from build123d import *

# Parameters (mm, degrees)
BOSS_EXTRUDE1_DEPTH = 58
SKETCH3_R           = 7.5
CUT_EXTRUDE1_DEPTH  = 107.60206377
CUT_EXTRUDE2_DEPTH  = 107.60206377
CUT_EXTRUDE3_DEPTH  = 107.60206377
SKETCH6_R           = 7
CUT_EXTRUDE4_DEPTH  = 107.60206377
CUT_EXTRUDE5_DEPTH  = 6
CUT_EXTRUDE6_DEPTH  = 4
CUT_EXTRUDE7_START  = -6
CUT_EXTRUDE7_DEPTH  = 6
CUT_EXTRUDE8_START  = -4
CUT_EXTRUDE8_DEPTH  = 4


with BuildPart() as part:
    # Sketch2 → Boss-Extrude1 (new body)
    with BuildSketch(Plane.XY):
        with BuildLine():
            Line((0, 0), (65, 0))
            Line((65, 0), (80, 9.029262631))
            Line((80, 9.029262631), (80, 31.339745962))
            Line((80, 31.339745962), (65, 40))
            Line((65, 40), (36.66060556, 40))
            ThreePointArc((36.66060556, 40), (16.66060556, 35.82575695), (0, 24))
            Line((0, 24), (0, 0))
        make_face()
    extrude(amount=-BOSS_EXTRUDE1_DEPTH)

    # Sketch3 → Cut-Extrude1 (cut, through all)
    with BuildSketch(Plane.XY):
        with Locations((34, 19)):
            Circle(SKETCH3_R)
    extrude(amount=-CUT_EXTRUDE1_DEPTH, mode=Mode.SUBTRACT)

    # Sketch4 → Cut-Extrude2 (cut, through all)
    with BuildSketch(Plane(origin=(0, 0, 0), x_dir=(1, 0, 0), z_dir=(0, 1, 0))):
        Polygon((65, 58), (80, 43), (80, 58), align=None)
        Polygon((80, 0), (80, 15), (65, 0), align=None)
    extrude(amount=CUT_EXTRUDE2_DEPTH, mode=Mode.SUBTRACT)

    # Sketch5 → Cut-Extrude3 (cut, through all)
    with BuildSketch(Plane.XZ):
        Polygon((0, -8), (0, -50), (16, -50), (16, -44), (54, -44), (54, -14), (16, -14), (16, -8), align=None)
    extrude(amount=-CUT_EXTRUDE3_DEPTH, mode=Mode.SUBTRACT)

    # Sketch6 → Cut-Extrude4 (cut, through all)
    with BuildSketch(Plane(origin=(80, 0, 0), x_dir=(0, 0, -1), z_dir=(1, 0, 0))):
        with Locations((29, 20)):
            Circle(SKETCH6_R)
    extrude(amount=-CUT_EXTRUDE4_DEPTH, mode=Mode.SUBTRACT)

    # Sketch8 → Cut-Extrude5 (cut)
    with BuildSketch(Plane.XY):
        with BuildLine():
            Line((1.466424222, 22.64), (0, 21.058823529))
            Line((0, 21.058823529), (0, 2))
            Line((0, 2), (63, 2))
            Line((63, 2), (63, 38))
            Line((63, 38), (36.66060556, 38))
            ThreePointArc((36.66060556, 38), (17.46060556, 33.992726672), (1.466424222, 22.64))
        make_face()
    extrude(amount=-CUT_EXTRUDE5_DEPTH, mode=Mode.SUBTRACT)

    # Sketch9 → Cut-Extrude6 (cut)
    with BuildSketch(Plane.XY.offset(-6)):
        with BuildLine():
            Line((18, 2), (63, 2))
            Line((63, 2), (63, 38))
            Line((63, 38), (36.66060556, 38))
            ThreePointArc((36.66060556, 38), (27.141221384, 37.046586751), (18, 34.224221872))
            Line((18, 34.224221872), (18, 2))
        make_face()
    extrude(amount=-CUT_EXTRUDE6_DEPTH, mode=Mode.SUBTRACT)

    # Sketch10 → Cut-Extrude7 (cut)
    with BuildSketch(Plane(origin=(0, 0, -58), x_dir=(-1, 0, 0), z_dir=(0, 0, -1)).offset(CUT_EXTRUDE7_START)):
        with BuildLine():
            Line((-1.466424222, 22.64), (0, 21.058823529))
            Line((0, 21.058823529), (0, 2))
            Line((0, 2), (-63, 2))
            Line((-63, 2), (-63, 38))
            Line((-63, 38), (-36.66060556, 38))
            ThreePointArc((-36.66060556, 38), (-17.46060556, 33.992726672), (-1.466424222, 22.64))
        make_face()
    extrude(amount=CUT_EXTRUDE7_DEPTH, mode=Mode.SUBTRACT)

    # Sketch11 → Cut-Extrude8 (cut)
    with BuildSketch(Plane(origin=(0, 0, -52), x_dir=(-1, 0, 0), z_dir=(0, 0, -1)).offset(CUT_EXTRUDE8_START)):
        with BuildLine():
            Line((-63, 38), (-63, 2))
            Line((-63, 2), (-18, 2))
            Line((-18, 2), (-18, 34.224221872))
            ThreePointArc((-18, 34.224221872), (-27.141221384, 37.046586751), (-36.66060556, 38))
            Line((-36.66060556, 38), (-63, 38))
        make_face()
    extrude(amount=CUT_EXTRUDE8_DEPTH, mode=Mode.SUBTRACT)


solid = part.part
Input: part model. Units: mm. Frame: model coordinates. A direction names the side the tool comes from. Coordinates: 2 decimals unless noted, no trailing zeros. Order: outer loops, then holes, each group sorted by start corner. A loop starts at its lowest first (then second) coordinate and runs counter-clockwise, first axis right, second up. Notation, with made-up numbers: M 63.5,41.5 L 122.5,41.5 A13 cw 122.5,53.5 Z; hole C 73,-34.75 d9. An arc over 180 degrees is marked long. One line per question, with ' | ' between items.
Item 1: Section D-D (y = 20). Give the number of separate pieces and of enclosed holes in the cut face, then the cut area to 3 significant figures.
Geometry results:
separate pieces: 4 | enclosed holes: 0 | area: 1,000 mm^2
Item 2: Draft query along X for faces 6 (the flat face through (9, 15, -52)), 7 (the flat face through (70.94, 36.57, -28.59)), 8 (the flat face through (38, 2, -5)), 9 (the flat face through (44, 20, -14)). Return one class per face: released by +X, released by -X, zero draft, split by the parting line, or undercut.
Geometry results:
face 6: undercut | face 7: released by +X | face 8: undercut | face 9: zero draft
Item 3: Section C-C (x = 51). Output: boundary loops of the cut face in (y, z), then the cut area to 3 significant figures.
Geometry results:
outline: M 0,-58 L 2,-58 L 2,-48 L 38,-48 L 38,-58 L 40,-58 L 40,-44 L 0,-44 Z; M 0,-14 L 40,-14 L 40,0 L 38,0 L 38,-10 L 2,-10 L 2,0 L 0,0 Z | area: 400 mm^2
Item 4: Reachability of faces 1 (the flat face through (50, 38, -53)), 2 (the flat face through (16, 18, -47)), 3 (the cylindrical face through (67.18, 13.79, -32.23)), 4 (the cylindrical face through (28.5, 24.1, -46)), 5 (the flat face through (45, 20, -10)) from +Z, -Z, +X, -X, +Y, -Y: full face, straight path, thin tool, end or side. Return the list, or none.
Geometry results:
face 1: -Z | face 2: -X, +Y, -Y | face 3: +X, -X | face 4: +Z, -Z | face 5: +Z
Item 5: Pin query (flat end, axial travel): pin 1 (1 mm diameter, centred on y = 10.5, z = -32, fed in from -X); pin 2 (3 mm diameter, centred on x = 19.5, z = -3, fed in from +Y); pin 3 (6 mm diameter, centred on x = 36, y = 18, fed in from -Z); pin 4 (8 mm diameter, centred on x = 23.5, z = -54.5, fed in from +Y). Return the tip coordinate at first contact, or that it passes through.
Geometry results:
pin 1: stops at x = 54 | pin 2: stops at y = 37.48 | pin 3: passes through | pin 4: stops at y = 39.15
Item 6: Section B-B (z = -29). Output: boundary loops of the cut face in (x, y), then the cut area to 3 significant figures.
Geometry results:
outline: M 54,0 L 65,0 L 80,9.03 L 80,13 L 54,13 Z; M 54,27 L 80,27 L 80,31.34 L 65,40 L 54,40 Z | area: 543 mm^2
Item 7: Section A-A (x = 61). Output: boundary loops of the cut face in (y, z).
Geometry results:
outline: M 0,-58 L 2,-58 L 2,-48 L 38,-48 L 38,-58 L 40,-58 L 40,0 L 38,0 L 38,-10 L 2,-10 L 2,0 L 0,0 Z; hole C 20,-29 d14
Item 8: Ray query, line 1 along Z through (x, y) = (48, 17); line 2 along Z through (x, y) = (7.5, 11); line 3 along Y through (x, z) = (60, -29). Return the intervals inside material, ascending.
Geometry results:
line 1: z = -48 to -44, -14 to -10 | line 2: z = -52 to -50, -8 to -6 | line 3: y = 0 to 13, 27 to 40
